Autodesk Inventor part; units mm, degrees
ref_plane "WorkPlane1" through (0, 0, 0) normal (0, 0, 1) x (1, 0, 0)
ref_plane "MSC_PF1" through (0, 0, 0) normal (1, 0, 0) x (0, 1, 0)
ref_plane "MSC_PT1" through (0, 0, 0) normal (0, 0, -1) x (-1, 0, 0)
ref_plane "WorkPlane1" through (0, 0, 0) normal (0, 0, 1) x (1, 0, 0)
sketch "Sketch1" plane through (0, 0, 0) normal (0, 0, 1) x (1, 0, 0)
  point P0 (0, 0)
sketch "Sketch2" plane through (0, 0, 0) normal (0, 0, 1) x (1, 0, 0)
  line L0 (-6.5, 3.7529) -> (-6.5, -3.7529)
  line L1 (0, 7.5054) -> (-6.5, 3.7529)
  line L2 (6.5, 3.7529) -> (0, 7.5054)
  line L3 (6.5, -3.7529) -> (6.5, 3.7529)
  line L4 (0, -7.5054) -> (6.5, -3.7529)
  line L5 (-6.5, -3.7529) -> (0, -7.5054)
  circle A0 centre (0, 0) radius 6.5 construction
  dimension "d1" = 13
  dimension "d29" = 0
  dimension "d30" = 0
extrude "Extrusion1" add sketch "Sketch2" along normal blind 5.3
sketch "Sketch3" plane through (0, 0, 0) normal (1, 0, 0) x (0, 1, 0)
  line L0 (6.5, 5.3) -> (7.6054, 5.3)
  line L1 (7.6054, 4.6618) -> (6.5, 5.3)
  line L2 (7.6054, 5.3) -> (7.6054, 4.6618)
  line L3 (0, -1.06) -> (0, 6.36)
  line L4 (7.5054, 0) -> (7.5054, 5.3)
  dimension "d25" = 0.1
  dimension "d26" = 0
  dimension "d27" = 60
  dimension "d28" = 6.5
revolve "Revolution1" cut sketch "Sketch3" angle 360 about axis through (0, 0, -10) along (0, 0, 1)
sketch "Sketch4" plane through (0, 0, 0) normal (1, 0, 0) x (0, 1, 0)
  line L0 (0, -60) -> (0, 0)
  line L1 (-4, -60) -> (0, -60)
  line L2 (-4, 0) -> (-4, -60)
  line L3 (0, 0) -> (-4, 0)
  line L4 (0, -60) -> (0, 0)
  line L5 (-4.8, 0) -> (0.8, 0)
  line L6 (0, -72) -> (0, 12)
  dimension "d18" = 4
  dimension "d20" = 60
  dimension "d33" = 0
  dimension "d34" = 0
revolve "Revolution2" add sketch "Sketch4" angle 360 about axis through (0, 0, -60) along (0, 0, -1)
chamfer "Chamfer1" distance 0.625 angle 45 1 edges at (0, 4, -60)
fillet "Fillet1" radius 0.4 1 edges at (0, 4, 0)
thread "Thread1"
ref_plane "MSC_PF1" through (0, 0, 0) normal (1, 0, 0) x (0, 1, 0)
ref_plane "MSC_PT1" through (0, 0, 0) normal (0, 0, -1) x (-1, 0, 0)
equation "\"d22\" = 0.5 * PTC"
equation "\"d23\" = 0.5 * PTC"
equation "\"d24\" = r"
equation "\"d1\" = ParS"
equation "\"d6\" = ParK"
equation "\"b\" = NLG - 2 * PTC"
equation "\"d28\" = 0.5 * ParS"
equation "\"d18\" = 0.5 * NND"
equation "\"d20\" = NLG"
equation "\"NND\" = 8"
equation "\"NLG\" = 60"
equation "\"PTC\" = 1.25"
equation "\"ParK\" = 5.3"
equation "\"ParS\" = 13"
equation "\"msp_es\" = 0.577367 * ParS"
equation "\"r\" = 0.4"
equation "\"THREADDIA\" = NND"
equation "\"K1\" = 3.45"
properties part number "DIN EN ISO 4018 - M8x60" material "Stainless Steel"
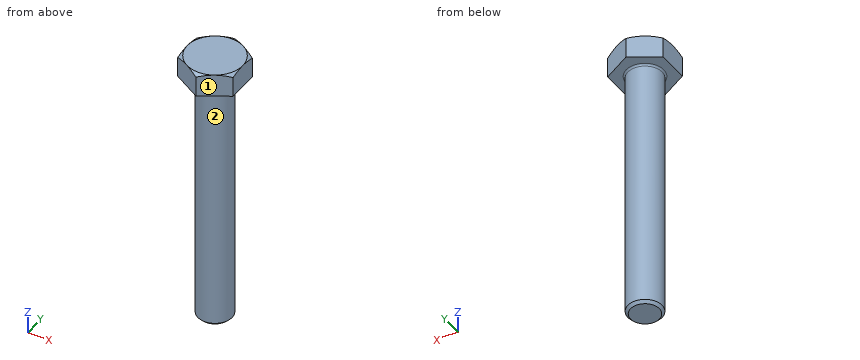
For this review, take the finished solid that the model builds, in its own axes (mm). Face numbers are marked on the shaded views. A direction names the side the tool comes from. Give positions to 0.01 mm unless a question says otherwise; leave off trailing zeros. Order: outer loops, then holes, each group sorted by start corner. A loop starts at its lowest first (then second) coordinate and runs counter-clockwise, first axis right, second up. Notation, with made-up numbers: M -7.75,23.5 L 42.25,23.5 A23 cw 42.25,40.5 Z; hole C -40,17 d10. An arc over 180 degrees is marked long. Answer in a Markdown table with one row per item. Add a question column.
(1) Wall thickness on probe 1 along Z at (x, y) = (5.25, -1); probe 2 along X at (y, z) = (-2.5, -48.5); probe 3 along Y at (x, z) = (3, -49.5): over which ranges is each line inside the solid? List them lowest first. Write a range as [from, to].
(2) For the marked faces 1 and 2, list the 3-axis set-ups (+Z, -Z, +X, -X, +Y, -Y) from which the entire face can be reached by the end or side of a thin tool; tool diameter is ignored.
(3) For pin 1 (5 mm diameter, centred on x = 2, z = -52, fed in from +Y); pin 2 (1 mm diameter, centred on x = -3.5, z = -9, fed in from +Y); pin 3 (4 mm diameter, centred on x = -3, z = -39, fed in from +Y), all flat-tipped, find the tip position at first contact; note any pin that passes through.
(4) Consider section A-A on z = -51.5. State the section outline as (x, y) points, and give its area (3 significant figures).
Evaluation:
| question | item | result |
|---|---|---|
| 1 | probe 1 | z = [0, 5.3] |
| 1 | probe 2 | x = [-3.12, 3.12] |
| 1 | probe 3 | y = [-2.65, 2.65] |
| 2 | face 1 | +Z, -Z, +X, -Y |
| 2 | face 2 | -Z |
| 3 | pin 1 | stops at y = 4 |
| 3 | pin 2 | stops at y = 2.65 |
| 3 | pin 3 | stops at y = 3.87 |
| 4 | outline | C 0,0 d8 |
| 4 | area | 50.3 mm^2 |
